Geometry: final body of the model. Coordinates: model frame, mm. Give positions to 0.01 mm unless a question says otherwise; leave off trailing zeros. Loops run counter-clockwise (first coordinate to the right, second up) from the corner with the lowest first, then second, coordinate; pieces in that order, holes last. Notation, with made-up numbers: M 5,26.25 L 55,26.25 A30 cw 55,51.25 Z; hole C 8,0.25 d11. An arc over 180 degrees is marked long. One line per question, with ' | ' between items. Start each with the question number.
from build123d import *

# Parameters (mm, degrees)
ESQUISSE1_W        = 55
ESQUISSE1_H        = 55
BOSS_EXTRU_1_DEPTH = 12
TROU_TARAUD_M121_D = 10.2
CHANFREIN1_SIZE    = 1


with BuildPart() as part:
    # Esquisse1 → Boss.-Extru.1 (new body)
    with BuildSketch(Plane(origin=(0, 0, 0), x_dir=(1, 0, 0), z_dir=(0, 1, 0))):
        with Locations((27.5, 27.5)):
            Rectangle(ESQUISSE1_W, ESQUISSE1_H)
    extrude(amount=BOSS_EXTRU_1_DEPTH)

    # Trou taraudé M121 (through all)
    with Locations(Plane.XZ):
        with Locations((27.5, -27.5)):
            Hole(TROU_TARAUD_M121_D / 2)

    # Chanfrein1
    chanfrein1_edges = [part.edges().sort_by_distance(p)[0] for p in [
        (55, 12, -27.5),
        (27.5, 12, -55),
        (32.6, 0, -27.5),
        (32.6, 12, -27.5),
        (0, 12, -27.5),
        (27.5, 0, -55),
        (55, 0, -27.5),
        (27.5, 0, 0),
        (0, 0, -27.5),
        (27.5, 12, 0),
        (0, 6, -55),
        (55, 6, -55),
        (55, 6, 0),
        (0, 6, 0),
    ]]
    chamfer(chanfrein1_edges, length=CHANFREIN1_SIZE)


solid = part.part
Q1. Section B-B, the plane z = -27.5. Output: boundary loops of the cut face in (x, y), plus the area to 3 significant figures.
Q2. Section A-A, the plane y = 6.5. Output: boundary loops of the cut face in (x, z), plus the area to 3 significant figures.
Q3. Material intervals for L1, parallel to Z at x = 27.5, y = 7.75; L2, parallel to Z at x = 27, y = 11.5; L3, parallel to X at y = 4.5, z = -25.5, sorted ascending.
Q4. Contact query for a flat-ended pin moving along its axis: pin 1 (6 mm diameter, centred on x = 27.5, z = -27.5, fed in from +Y). Output: stop coordinate, or through.
Q5. Draft query along X for faces 1 (the flat face through (0, 6, -27)), 2 (the flat face through (27, 6, 0)), 3 (the cylindrical face through (31.55, 6.07, -30.6)), 4 (the flat face through (55, 6, -27)). Return one class per face: released by +X, released by -X, zero draft, split by the parting line, or undercut.
Q6. Section C-C, the plane x = 27.5. Output: boundary loops of the cut face in (y, z).
Model answer:
1) outline: M 0,1 L 1,0 L 21.4,0 L 22.4,1 L 22.4,11 L 21.4,12 L 1,12 L 0,11 Z; M 32.6,1 L 33.6,0 L 54,0 L 55,1 L 55,11 L 54,12 L 33.6,12 L 32.6,11 Z | area: 534 mm^2
2) outline: M 0,-54 L 1,-55 L 54,-55 L 55,-54 L 55,-1 L 54,0 L 1,0 L 0,-1 Z; hole C 27.5,-27.5 d10.2 | area: 2,940 mm^2
3) L1: z = -55 to -32.6, -22.4 to 0 | L2: z = -54.5 to -33.08, -21.92 to -0.5 | L3: x = 0 to 22.81, 32.19 to 55
4) pin 1: passes through
5) face 1: released by -X | face 2: zero draft | face 3: undercut | face 4: released by +X
6) outline: M 0,-54 L 1,-55 L 11,-55 L 12,-54 L 12,-33.6 L 11,-32.6 L 1,-32.6 L 0,-33.6 Z; M 0,-21.4 L 1,-22.4 L 11,-22.4 L 12,-21.4 L 12,-1 L 11,0 L 1,0 L 0,-1 Z
